Geometry: see drawing. Coordinates: mm, zero at the bounding-box minimum. A direction names the side the tool comes from. Round coordinates to 2 decimals unless told otherwise and drop trailing zeros. Loops run counter-clockwise (first coordinate to the right, second up) from the corner with the lowest first, then second, coordinate; pieces in that order, holes last. Notation, with made-up numbers: (-34, 74.5) -> (-15, 74.5) arc R10 ccw to (-15, 78.5) -> close; hole circle Ø10 at (87.5, -15). An arc over 180 degrees is marked (long way). Write item = value, one per line.
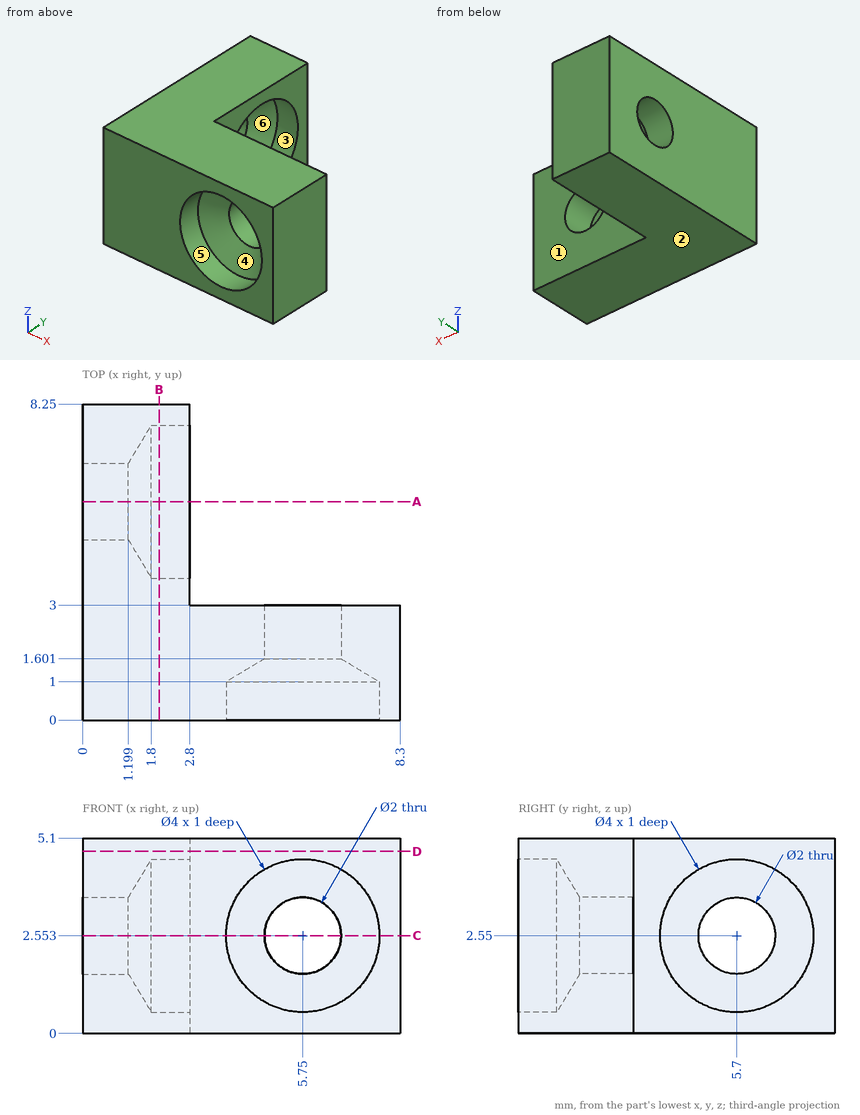
1. Contact query for flat-ended pins moving along their axis: pin 1 Ø1.5 at (y, z) = (6, 1.5) entering from +X (1 decimal); pin 2 Ø2.5 at (y, z) = (5.7, 2.55) entering from +X; pin 3 Ø2.5 at (x, z) = (5.75, 2.55) entering from -Y; pin 4 Ø1.5 at (x, y) = (3, 6) entering from -Z. Output: stop coordinate, or through.
Evaluation:
pin_1 = 1.7
pin_2 = 1.35
pin_3 = 1.45
pin_4 = 0
2. Set-up query: the marked faces 1 and 2. Return all of +Z, -Z, +X, -X, +Y, -Y with unobstructed straight access to the full face (end or side cutting, diameter ignored); none if empty.
Evaluation:
face_1 = +Z, -Z, +X, +Y
face_2 = -Z, +X, -X, +Y, -Y
3. Section query B-B (x = 2). Return the cut outline in (y, z).
Evaluation:
outline = (0, 0) -> (8.25, 0) -> (8.25, 5.1) -> (0, 5.1) -> close; hole circle Ø4 at (5.7, 2.55)
4. Section query C-C (z = 2.55). Give the number of separate pieces and of enclosed holes in the cut face, then the cut area to 3 significant figures.
Evaluation:
separate_pieces = 3
enclosed_holes = 0
area = 22.8 mm²
5. Section query A-A (y = 5.7). Return the cut outline in (x, z).
Evaluation:
outline = (0, 0) -> (2.8, 0) -> (2.8, 0.55) -> (1.8, 0.55) -> (1.2, 1.55) -> (0, 1.55) -> close; (0, 3.55) -> (1.2, 3.55) -> (1.8, 4.55) -> (2.8, 4.55) -> (2.8, 5.1) -> (0, 5.1) -> close
6. Section query D-D (z = 4.75). Return the cut outline in (x, y).
Evaluation:
outline = (0, 0) -> (8.3, 0) -> (8.3, 3) -> (2.8, 3) -> (2.8, 8.25) -> (0, 8.25) -> close
7. Line query: probe 1 along Y at (x, z) = (0.5, 2.55); probe 2 along Z at (x, y) = (0.65, 5.7); probe 3 along Y at (x, z) = (2.1, 2.55). Output: solid intervals per line, ascending. Write a range as from..to.
Evaluation:
probe_1 = 0..4.7, 6.7..8.25
probe_2 = 0..1.55, 3.55..5.1
probe_3 = 0..3.7, 7.7..8.25
8. Mould query, pull axis Y, two halves, no side actions, for the marked faces 3, 4, 5 and 6. Classes: released by +Y, released by -Y, zero draft, split by the parting line, or undercut.
Evaluation:
face_3 = undercut
face_4 = released by -Y
face_5 = zero draft
face_6 = undercut
